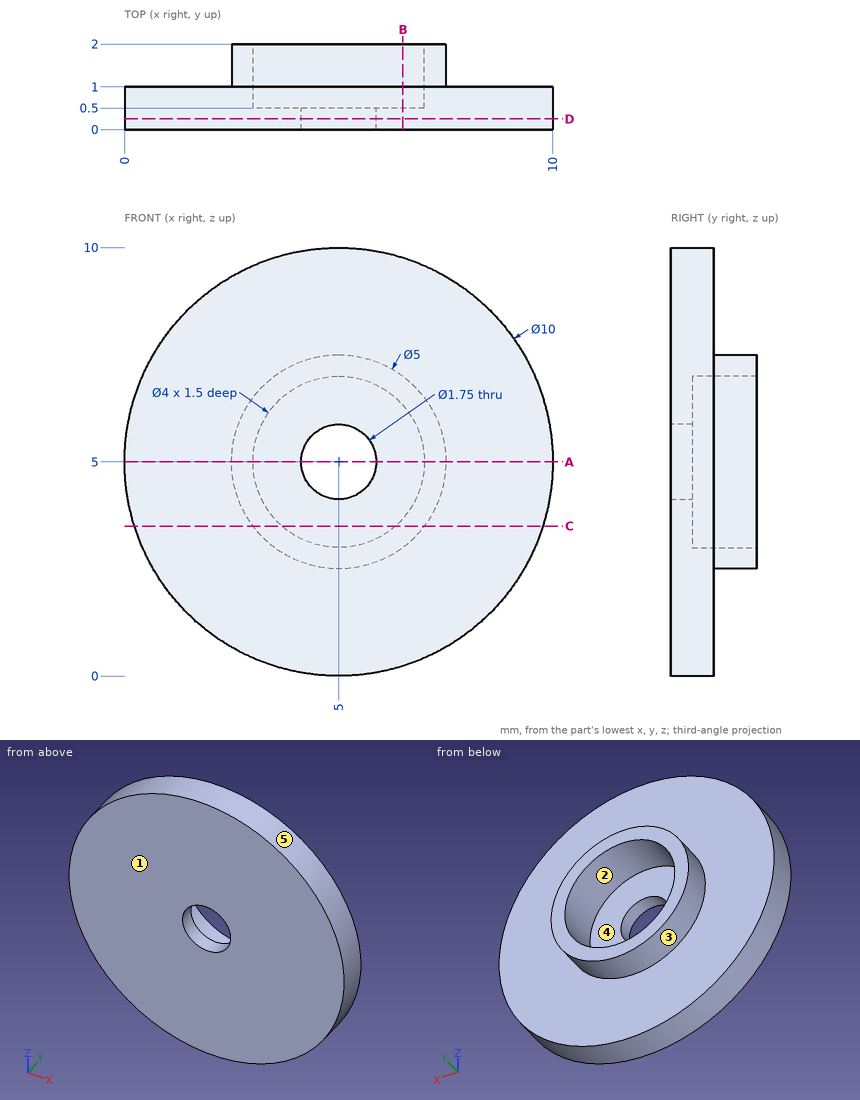
Print and shaded views of the part. All mm, measured from the part's lowest x, y and z. A direction names the side the tool comes from. Round coordinates to 2 decimals unless told otherwise and drop trailing zeros. Order: outer loops, then holes, each group sorted by start corner. A loop starts at its lowest first (then second) coordinate and runs counter-clockwise, first axis right, second up.
Q1. Slice it at A-A (z = 5). Write the cut outline in (x, y) (3 decimals).
Q2. Slice it at C-C (z = 3.5). Write the cut outline in (x, y), and give its area (3 significant figures).
Q3. Which spindle directions (+Z, -Z, +X, -X, +Y, -Y) get a long thin tool onto all of the face, cutting with end or side? Do the marked faces 4 and 5. Say none if no direction does.
Q4. Slice it at D-D (y = 0.25). Write the cut outline in (x, z) (3 decimals), and give its area (3 significant figures).
Q5. Drop flat-ended pins along their axis: pin 1 (1 mm diameter, centred on y = 0.5, z = 6.5, fed in from +X); pin 2 (1.2 mm diameter, centred on x = 5, z = 5, fed in from +Y). Give the stop position or say it passes through.
Q6. Slice it at B-B (x = 6.5). Write the cut outline in (y, z), and give its area (3 significant figures).
Q7. Two-plate mould, pull along X, no slides. Class the marked faces 1, 2 and 3: pulls with the +X half, pulls with the -X half, needs draft (parallel to the pull), parting line crosses it, or undercut.
Q8. Wall check: L1, parallel to X at y = 1.5, z = 5; L2, parallel to X at y = 0.2, z = 5 (3 decimals); L3, parallel to Y at x = 1.75, z = 3. Give the ranges that are in metal, low to high.
Results below:
1. outline: (0, 0) - (4.125, 0) - (4.125, 0.5) - (3, 0.5) - (3, 2) - (2.5, 2) - (2.5, 1) - (0, 1) - close; (5.875, 0) - (10, 0) - (10, 1) - (7.5, 1) - (7.5, 2) - (7, 2) - (7, 0.5) - (5.875, 0.5) - close
2. outline: (0.23, 0) - (9.77, 0) - (9.77, 1) - (7, 1) - (7, 2) - (6.32, 2) - (6.32, 0.5) - (3.68, 0.5) - (3.68, 2) - (3, 2) - (3, 1) - (0.23, 1) - close
2. area: 9.57 mm2
3. face 4: +Y
3. face 5: +Y, -Y
4. outline: circle Ø10 at (5, 5); hole circle Ø1.75 at (5, 5)
4. area: 76.1 mm2
5. pin 1: stops at x = 9.9
5. pin 2: passes through
6. outline: (0, 0.23) - (1, 0.23) - (1, 3) - (2, 3) - (2, 3.68) - (0.5, 3.68) - (0.5, 6.32) - (2, 6.32) - (2, 7) - (1, 7) - (1, 9.77) - (0, 9.77) - close
6. area: 9.57 mm2
7. face 1: needs draft
7. face 2: undercut
7. face 3: parting line crosses it
8. L1: x = 2.5 to 3, 7 to 7.5
8. L2: x = 0 to 4.125, 5.875 to 10
8. L3: y = 0 to 1
